The model under review builds one solid part; all positions refer to its coordinate system, in mm. Face numbers are marked on the shaded views. A direction names the side the tool comes from. Coordinates: 2 decimals unless noted, no trailing zeros. Order: outer loops, then holes, each group sorted by start corner. A loop starts at its lowest first (then second) coordinate and runs counter-clockwise, first axis right, second up. Notation, with made-up numbers: (75.5, -9.75) -> (90.5, -9.75) arc R27 cw to (90.5, 25.25) -> close; hole circle Ø6 at (51.25, -4). An arc over 180 degrees is marked (long way). Put each result on its own line as item: value.
from build123d import *

# Parameters (mm, degrees)
BOSS_EXTRUDE1_DEPTH      = 21
BOSS_EXTRUDE1_DEPTH_BACK = 21
SKETCH1_W                = 10
SKETCH1_H                = 20
SKETCH1_W_2              = 8
SKETCH1_H_2              = 18
SKETCH2_R                = 2.5
CUT_EXTRUDE1_DEPTH       = 20


with BuildPart() as part:
    # Sketch1 → Boss-Extrude1 (new, two sides: drawn at the far end of the back side and taken through both)
    with BuildSketch(Plane(origin=(0, 0, 0), x_dir=(0, 0, -1), z_dir=(1, 0, 0)).offset(-BOSS_EXTRUDE1_DEPTH_BACK)):
        Rectangle(SKETCH1_W, SKETCH1_H)
        Rectangle(SKETCH1_W_2, SKETCH1_H_2, mode=Mode.SUBTRACT)
    extrude(amount=BOSS_EXTRUDE1_DEPTH + BOSS_EXTRUDE1_DEPTH_BACK)

    # Sketch2 → Cut-Extrude1 (cut)
    with BuildSketch(Plane(origin=(0, 10, 0), x_dir=(1, 0, 0), z_dir=(0, 1, 0))):
        with Locations(Location((-16, 0, 0), (0, 0, 270))):
            Circle(SKETCH2_R)
        with Locations(Location((16, 0, 0), (0, 0, 270))):
            Circle(SKETCH2_R)
    extrude(amount=-CUT_EXTRUDE1_DEPTH, mode=Mode.SUBTRACT)


solid = part.part
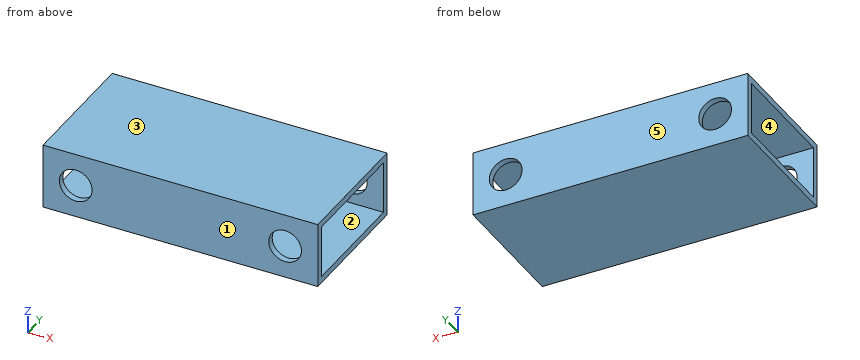
Item 1: Mouldability with a two-part tool opening along Y and no side actions: class the marked faces 1, 2 and 3 as +Y half, -Y half, draft (parallel to the pull), parting line (faces both ways), or undercut.
Answers below:
face 1: -Y half
face 2: undercut
face 3: draft
Item 2: For the marked faces 4 and 5, list the 3-axis set-ups (+Z, -Z, +X, -X, +Y, -Y) from which the entire face can be reached by the end or side of a thin tool; tool diameter is ignored.
Answers below:
face 4: +X, -X
face 5: +Z, -Z, +X, -X, +Y
Item 3: Consider section D-D on z = 0. Write out the cut boundary in (x, y), and give its area (3 significant figures).
Answers below:
outline: (-21, -10) -> (-18.5, -10) -> (-18.5, -9) -> (-21, -9) -> close; (-21, 9) -> (-18.5, 9) -> (-18.5, 10) -> (-21, 10) -> close; (-13.5, -10) -> (13.5, -10) -> (13.5, -9) -> (-13.5, -9) -> close; (-13.5, 9) -> (13.5, 9) -> (13.5, 10) -> (-13.5, 10) -> close; (18.5, -10) -> (21, -10) -> (21, -9) -> (18.5, -9) -> close; (18.5, 9) -> (21, 9) -> (21, 10) -> (18.5, 10) -> close
area: 64.0 mm^2
Item 4: Consider section C-C on x = -16. Write out the cut boundary in (y, z).
Answers below:
outline: (-10, -5) -> (10, -5) -> (10, -2.5) -> (9, -2.5) -> (9, -4) -> (-9, -4) -> (-9, -2.5) -> (-10, -2.5) -> close; (-10, 2.5) -> (-9, 2.5) -> (-9, 4) -> (9, 4) -> (9, 2.5) -> (10, 2.5) -> (10, 5) -> (-10, 5) -> close
Item 5: Consider section A-A on z = -3. Write out the cut boundary in (x, y).
Answers below:
outline: (-21, -10) -> (21, -10) -> (21, -9) -> (-21, -9) -> close; (-21, 9) -> (21, 9) -> (21, 10) -> (-21, 10) -> close
Item 6: For line 1 (X direction, y = -9.3, z = 0); line 2 (Z direction, x = -5.5, y = 3.5); line 3 (Y direction, x = -11, z = 2.75), list the stretches that pass through material, from the lowest coordinate up. Write a range as from..to.
Answers below:
line 1: -21..-18.5, -13.5..13.5, 18.5..21
line 2: -5..-4, 4..5
line 3: -10..-9, 9..10
Item 7: For pin 1 Ø4.5 at (x, z) = (16, 0) entering from +Y, flat-tipped, find the tip position at first contact; note if it passes through.
Answers below:
pin 1: through
Item 8: Consider section B-B on y = -5.5. Write out the cut boundary in (x, z).
Answers below:
outline: (-21, -5) -> (21, -5) -> (21, -4) -> (-21, -4) -> close; (-21, 4) -> (21, 4) -> (21, 5) -> (-21, 5) -> close
